Autodesk Inventor part; units mm, degrees
ref_plane "YZ Plane" through (0, 0, 0) normal (1, 0, 0) x (0, 1, 0)
ref_plane "XZ Plane" through (0, 0, 0) normal (0, 1, 0) x (-1, 0, 0)
ref_plane "XY Plane" through (0, 0, 0) normal (0, 0, 1) x (1, 0, 0)
sketch "Sketch1" plane through (0, 0, 0) normal (0, 1, 0) x (-1, 0, 0)
  circle A0 centre (0, 0) radius 20
  circle A1 centre (0, 0) radius 15
  line L0 (-0.5, -14.9917) -> (-0.5, -19.9937)
  line L1 (0.5, -19.9937) -> (0.5, -14.9917)
  line L2 (0, -28) -> (0, 28)
  circle A2 centre (0, 0) radius 15.7
  point P0 (-0.5, -15.692)
  point P1 (0.5, -15.692)
  dimension "d0" = 40
  dimension "d1" = 5
  dimension "d2" = 1
  dimension "d5" = 4.3
extrude "Extrusion1" add sketch "Sketch1" along normal blind 3.25 contours L1 A2 L2 A0 | L2 A2 L0 A0 picked at (18.3995, 1.4835) picked at (-2.823, 18.227)
ref_plane "Work Plane1" through (0, 0, -14.9917) normal (1, 0, 0) x (0, 0, -1)
properties part number "Test_Radiator_Disc"
Can you work these out from the model? Positions are in its coordinate system, mm. Coordinates: 2 decimals unless noted, no trailing zeros. Write each loop counter-clockwise with the first axis right and the second up, starting at its lowest first coordinate (ties: lowest second). Pieces come first, ordered by that corner, then holes. Notation, with made-up numbers: (6.25, 12.25) - (40.25, 12.25) arc R35 ccw to (40.25, 51.25) - close; hole circle Ø5 at (34, -8.5). An arc over 180 degrees is marked (long way). Return JSON: item names as keys, results as strings.
Q1. If we section it at C-C (y = 2.4): Please give me the cut outline in (x, z), then the cut area to 3 significant figures.
Computed values:
{"outline": "(-0.5, -19.99) - (-0.5, -15.69) arc R15.7 cw (long way) to (0.5, -15.69) - (0.5, -19.99) arc R20 ccw (long way) to start", "area": "478 mm2"}
Q2. Please list where these lines run through material, in increasing order: L1, parallel to X at y = 1.8, z = 0; L2, parallel to Z at x = -14, y = 1.9; L3, parallel to X at y = 1.45, z = 4.5. Write a range as from..to.
Computed values:
{"L1": "x = -20..-15.7, 15.7..20", "L2": "z = -14.28..-7.11, 7.11..14.28", "L3": "x = -19.49..-15.04, 15.04..19.49"}
Q3. If we section it at A-A (x = -10): Please give me the cut outline in (y, z).
Computed values:
{"outline": "(0, -17.32) - (3.25, -17.32) - (3.25, -12.1) - (0, -12.1) - close; (0, 12.1) - (3.25, 12.1) - (3.25, 17.32) - (0, 17.32) - close"}
Q4. If we section it at D-D (x = 0): Please give me the cut outline in (y, z).
Computed values:
{"outline": "(0, 15.7) - (3.25, 15.7) - (3.25, 20) - (0, 20) - close"}
Q5. I'm going to push flat-ended pins straight in: pin 1 Ø10 at (x, z) = (-5, -4) entering from +Y; pin 2 Ø1.6 at (y, z) = (1, -18.5) entering from -X. Where does each tip first touch, or does it pass through?
Computed values:
{"pin 1": "passes through", "pin 2": "stops at x = -9.31"}
Q6. Thinking about a two-plate mould opening in X: for faces 1 (the flat face through (0.5, 2, -18)), 2 (the flat face through (-0.5, 2, -18)), 3 (the flat face through (10.5, 0, 11.9)), which applies, +X half, -X half, draft (parallel to the pull), parting line (faces both ways), or undercut?
Computed values:
{"face 1": "undercut", "face 2": "undercut", "face 3": "draft"}
Q7. If we section it at B-B (z = -4): Please give me the cut outline in (x, y).
Computed values:
{"outline": "(-19.6, 0) - (-15.18, 0) - (-15.18, 3.25) - (-19.6, 3.25) - close; (15.18, 0) - (19.6, 0) - (19.6, 3.25) - (15.18, 3.25) - close"}
